Can you work these out from the model? Positions are in its coordinate system, mm. A direction names the side the tool comes from. Give positions to 0.01 mm unless a question says otherwise; leave off trailing zeros. Write each loop counter-clockwise with the first axis right and the second up, starting at its lowest first coordinate (ties: lowest second). Pieces come first, ordered by that corner, then holes. Notation, with made-up numbers: (-34, 65) -> (10, 65) arc R23 cw to (10, 74) -> close; hole circle Ø7 at (37.5, -32). An arc over 180 degrees is marked (long way). One line per item, written item: value.
from build123d import *

# Parameters (mm, degrees)
SKETCH1_R          = 3.9624
EXTRUDE3_DEPTH     = 1.8288
SKETCH4_W          = 15.875
SKETCH4_H          = 2.0828
CHAMFER1_SIZE      = 0.5953125
SKETCH26_R         = 1.0414
EXTRUDE8_DEPTH     = 1.8288
CUT_EXTRUDE3_REACH = 18.835
CIRPATTERN1_COUNT  = 4
DRAFT2_ANGLE       = 5


# Read off the part's stored shape, not the designer's step: Extrude10, Draft1
with BuildPart() as part:
    # Sketch1 → Extrude3 (new body)
    with BuildSketch(Plane.XY):
        Circle(SKETCH1_R)
    extrude(amount=EXTRUDE3_DEPTH)

    # Sketch11 → Cut-Revolve3 (revolve, cut)
    with BuildSketch(Plane(origin=(0, 0, 0), x_dir=(0, 0, -1), z_dir=(1, 0, 0)), mode=Mode.PRIVATE) as cut_revolve3_sk:
        Polygon((0, 1.78292103), (-1.8288, 3.9624), (0, 3.9624), align=None)
    revolve(cut_revolve3_sk.sketch.rotate(Axis((0, 0, -0.441444004), (0, 0, 1)), 90), axis=Axis((0, 0, -0.441444004), (0, 0, 1)), mode=Mode.SUBTRACT)

    # Extrude10 outline → Extrude10 (revolve)
    with BuildSketch(Plane.XZ):
        Polygon((2.0828, 0), (2.0828, 0.251628333), (1.78292103, 0.251628333), (1.78292103, 0), (0, 0), (0, -2.0828), align=None)
    revolve(axis=Axis((0, 0, 0), (0, 0, 1)))



with BuildPart() as body_2:
    # Sketch4 → Revolve1 (revolve)
    with BuildSketch(Plane(origin=(0, 0, 0), x_dir=(0, 0, -1), z_dir=(1, 0, 0)), mode=Mode.PRIVATE) as revolve1_sk:
        with Locations((6.1087, 1.0414)):
            Rectangle(SKETCH4_W, SKETCH4_H)
    revolve(revolve1_sk.sketch.rotate(Axis((0, 0, 1.8288), (0, 0, -1)), 180), axis=Axis((0, 0, 1.8288), (0, 0, -1)))

    # Chamfer1
    chamfer1_edges = [body_2.edges().sort_by_distance(p)[0] for p in [
        (0, 2.0828, -14.0462),
    ]]
    chamfer(chamfer1_edges, length=CHAMFER1_SIZE)


with BuildPart() as part_1:
    add(part.part)

    add(body_2.part)  # Extrude8 merges body 2
    # Sketch26 → Extrude8 (add)
    with BuildSketch(Plane.XY.offset(1.8288)):
        Circle(SKETCH26_R)
    extrude(amount=-EXTRUDE8_DEPTH)

    # Cut-Extrude3: up to this cone (the profile starts inside it)
    cut_extrude3_end = Plane(origin=(0, 0, 1.8288), z_dir=(0, 0, 1)).offset(-2.462756405) * Cone(1.192e-06, 29.475352474, 24.732756389, align=(Align.CENTER, Align.CENTER, Align.MIN), mode=Mode.PRIVATE)
    # Sketch12 → Cut-Extrude3 (cut, up to the surface)
    with BuildSketch(Plane.XY.offset(1.8288), mode=Mode.PRIVATE) as cut_extrude3_sk1:
        with BuildLine():
            Line((2.588228842, 0.52832), (1.558274421, 0.52832))
            Line((1.558274421, 0.52832), (0.829986666, 0.829986666))
            Line((0.829986666, 0.829986666), (0.52832, 1.558274421))
            Line((0.52832, 1.558274421), (0.52832, 2.588228842))
            ThreePointArc((0.52832, 2.588228842), (0.265504474, 2.628223342), (0, 2.6416))
            Line((0, 2.6416), (0, 0))
            Line((0, 0), (2.6416, 0))
            ThreePointArc((2.6416, 0), (2.628223342, 0.265504474), (2.588228842, 0.52832))
        make_face()
    cut_extrude3_tool1 = extrude(cut_extrude3_sk1.sketch, amount=-CUT_EXTRUDE3_REACH, mode=Mode.PRIVATE) & cut_extrude3_end
    cut_extrude3 = cut_extrude3_tool1.solids().sort_by_distance((2.591055, 0.26175, 1.8288))[0]
    add(cut_extrude3, mode=Mode.SUBTRACT)

    # CirPattern1: Cut-Extrude3 ×4 about axis
    cirpattern1_axis = Axis((0, 0, 0), (0, 0, 1))
    for i in range(1, CIRPATTERN1_COUNT):
        add(cut_extrude3.rotate(cirpattern1_axis, i * 360 / CIRPATTERN1_COUNT), mode=Mode.SUBTRACT)

    # Draft1 outline → Draft1 (revolve)
    with BuildSketch(Plane.XZ):
        Polygon((2.6416, 1.8288), (2.556499421, 1.511200317), (2.6416, 1.511200317), align=None)
    revolve(axis=Axis((0, 0, 0), (0, 0, 1)))

    # Draft2
    draft2_faces = [part_1.faces().sort_by_distance(p)[0] for p in [
        (0.52832, 1.956108767, 1.448849015),
        (0.686884975, 1.175464708, 1.173602986),
        (1.175464708, 0.686884975, 1.173602986),
        (1.956108767, 0.52832, 1.448849015),
        (1.956108767, -0.52832, 1.448849015),
        (1.175464708, -0.686884975, 1.173602986),
        (0.686884975, -1.175464708, 1.173602986),
        (0.52832, -1.956108767, 1.448849015),
        (-0.52832, -1.956108767, 1.448849015),
        (-0.686884975, -1.175464708, 1.173602986),
        (-1.175464708, -0.686884975, 1.173602986),
        (-1.956108767, -0.52832, 1.448849015),
        (-1.956108767, 0.52832, 1.448849015),
        (-1.175464708, 0.686884975, 1.173602986),
        (-0.686884975, 1.175464708, 1.173602986),
        (-0.52832, 1.956108767, 1.448849015),
    ]]
    draft(draft2_faces, Plane(origin=(0, 2.0828, 1.8288), x_dir=(0, 1, 0), z_dir=(0, 0, 1)), DRAFT2_ANGLE)


solid = part_1.part
1) I need wall thicknesses on L1, parallel to Y at x = 0, z = -3.5; L2, parallel to Y at x = 1.5, z = -1.75. Which ranges of each line are inside material? Lowest first, please.
Answer list:
L1: y = -2.08 to 2.08
L2: y = -1.45 to 1.45
2) For faces 1 (the face through (0, 0, -14.046)), 2 (the face through (1.144, -0.625, 1.037)), which set-ups out of +Z, -Z, +X, -X, +Y, -Y let a thin tool reach every point of the face, with its end or its side?
Answer list:
face 1: -Z, +X, -X, +Y, -Y
face 2: +Z
3) If we section it at B-B (z = -4.5): Write out the boundary of the cut face in (x, y), and give its area (3 significant figures).
Answer list:
outline: circle Ø4.17 at (0, 0)
area: 13.6 mm^2
4) We'd pull the mould along X, two halves only. Please class faces 3 (the face through (1, 1, 1.829)), 4 (the face through (-1.94, 0.49, 1.4)), 5 (the face through (-2.1, -0.66, 0.35)): released by +X, released by -X, zero draft, split by the parting line, or undercut.
Answer list:
face 3: zero draft
face 4: undercut
face 5: split by the parting line
5) Will these pins go through, and if not, where does the flat tip stop? pin 1 (4 mm diameter, centred on y = 0, z = -1.5, fed in from +X); pin 2 (1.5 mm diameter, centred on y = -1, z = -7.5, fed in from -X); pin 3 (3 mm diameter, centred on x = 1.5, z = -5, fed in from -Y).
Answer list:
pin 1: stops at x = 2.38
pin 2: stops at x = -2.07
pin 3: stops at y = -2.08
6) If we section it at A-A (z = 1): Write out the boundary of the cut face in (x, y).
Answer list:
outline: circle Ø5.95 at (0, 0); hole (-1.89, -0.46) -> (-1.54, -0.46) -> (-0.77, -0.77) -> (-0.46, -1.54) -> (-0.46, -1.89) arc R1.95 ccw to (0.46, -1.89) -> (0.46, -1.54) -> (0.77, -0.77) -> (1.54, -0.46) -> (1.89, -0.46) arc R1.95 ccw to (1.89, 0.46) -> (1.54, 0.46) -> (0.77, 0.77) -> (0.46, 1.54) -> (0.46, 1.89) arc R1.95 ccw to (-0.46, 1.89) -> (-0.46, 1.54) -> (-0.77, 0.77) -> (-1.54, 0.46) -> (-1.89, 0.46) arc R1.95 ccw to start
